from build123d import *

# Parameters (mm, degrees)
F1_DEPTH = 15
F2_R     = 10
F3_DEPTH = 25


with BuildPart() as f1:
    # F0 (on Front) → F1 (new body)
    with BuildSketch(Plane.XZ):
        with BuildLine():
            ThreePointArc((-20, 0), (0, -20), (20, 0))
            ThreePointArc((20, 0), (0, 20), (-20, 0))
        make_face()
        with BuildLine():
            ThreePointArc((-20, 0), (0, 20), (20, 0))
            Line((20, 0), (20, 140))
            ThreePointArc((20, 140), (0, 120), (-20, 140))
            Line((-20, 140), (-20, 0))
        make_face()
        with BuildLine():
            ThreePointArc((-20, 140), (0, 120), (20, 140))
            ThreePointArc((20, 140), (0, 160), (-20, 140))
        make_face()
    extrude(amount=F1_DEPTH)

    # F2 (on face) → F3 (cut)
    with BuildSketch(Plane.XZ.offset(15)):
        with Locations((0, 140)):
            Circle(F2_R)
        Circle(F2_R)
    extrude(amount=-F3_DEPTH, mode=Mode.SUBTRACT)


solid = f1.part
Can you work these out from the model? Positions are in its coordinate system, mm. Coordinates: 2 decimals unless noted, no trailing zeros. Loops run counter-clockwise (first coordinate to the right, second up) from the corner with the lowest first, then second, coordinate; pieces in that order, holes last. Notation, with made-up numbers: M 84.25,67.5 L 102.25,67.5 A21 ccw 102.25,71.5 Z; hole C -27.5,24.25 d5. An arc over 180 degrees is marked long. Answer as CSV lines item,"result". Start each with the question number.
1. For pin 1 Ø2 at (x, y) = (-1, -5.5) entering from -Z; pin 2 Ø3 at (x, y) = (-4.5, -6.5) entering from +Z; pin 3 Ø18 at (x, z) = (0, 0) entering from +Y, each with a flat end and sliding along its axis, tell me the tip position at first contact or that it passes through.
2. Suppose I cut it at A-A, the plane x = 0. List the corners of the cut face in (y, z) for me, plus the area to 3 significant figures.
3. Suppose I cut it at D-D, the plane z = -5.5. List the corners of the cut face in (x, y) for me.
4. Suppose I cut it at C-C, the plane y = -7.75. List the corners of the cut face in (x, z) for me, plus the area to 3 significant figures.
5. If I drill on probe 1 along Z at (x, y) = (0, -5.5); probe 2 along Z at (x, y) = (1.5, -10.5); probe 3 along X at (y, z) = (-3, 6.5), over which ranges is the centre line in solid material (lowest first)? Write a range as [from, to].
6. Suppose I cut it at B-B, the plane z = 136. List the corners of the cut face in (x, y) for me.
7. Thinking about a two-plate mould opening in X: for faces 1 (the face through (-2.17, -7.6, 130.24)), 2 (the face through (20, -7, 69)), 3 (the face through (0, -7, 160)), 4 (the face through (0, 0, 71)), which applies, +X half, -X half, draft (parallel to the pull), parting line (faces both ways), or undercut?
Output:
1,pin 1,"stops at z = -20"
1,pin 2,"stops at z = 159.77"
1,pin 3,"passes through"
2,outline,"M -15,-20 L 0,-20 L 0,-10 L -15,-10 Z; M -15,10 L 0,10 L 0,130 L -15,130 Z; M -15,150 L 0,150 L 0,160 L -15,160 Z"
2,area,"2,100 mm^2"
3,outline,"M -19.23,-15 L -8.35,-15 L -8.35,0 L -19.23,0 Z; M 8.35,-15 L 19.23,-15 L 19.23,0 L 8.35,0 Z"
4,outline,"M -20,0 A20 ccw 20,0 L 20,140 A20 ccw -20,140 Z; hole C 0,0 d20; hole C 0,140 d20"
4,area,"6,230 mm^2"
5,probe 1,"z = [-20, -10], [10, 130], [150, 160]"
5,probe 2,"z = [-19.94, -9.89], [9.89, 130.11], [149.89, 159.94]"
5,probe 3,"x = [-20, -7.6], [7.6, 20]"
6,outline,"M -20,-15 L -9.17,-15 L -9.17,0 L -20,0 Z; M 9.17,-15 L 20,-15 L 20,0 L 9.17,0 Z"
7,face 1,"undercut"
7,face 2,"+X half"
7,face 3,"parting line"
7,face 4,"draft"
